```python
from build123d import *

# Parameters (mm, degrees)
AUFSATZ_LINEAR_AUSTRAGEN1_DEPTH = 15
M5_GEWINDEBOHRUNG1_D            = 4.2
M5_GEWINDEBOHRUNG1_DEPTH        = 14
M5_GEWINDEBOHRUNG1_TIP          = 1.2618073
SKIZZE4_W                       = 45
SKIZZE4_H                       = 51.25
SCHNITT_LINEAR_AUSTRAGEN1_DEPTH = 8
VERRUNDUNG1_R                   = 5
VERRUNDUNG2_R                   = 5
M3_GEWINDEBOHRUNG1_D            = 2.5
M3_GEWINDEBOHRUNG1_DEPTH        = 8.5
M3_GEWINDEBOHRUNG1_TIP          = 0.751075774


with BuildPart() as part:
    # Skizze1 → Aufsatz-Linear austragen1 (new body)
    with BuildSketch(Plane.XY):
        with BuildLine():
            Line((100.5, 0), (115, 0))
            Line((115, 0), (115, 48))
            Line((115, 48), (78.75, 84.25))
            Line((78.75, 84.25), (36.25, 84.25))
            Line((36.25, 84.25), (0, 48))
            Line((0, 48), (0, 0))
            Line((0, 0), (14.5, 0))
            Line((14.5, 0), (14.5, 23.138097353))
            ThreePointArc((14.5, 23.138097353), (14.050252532, 33.449747468), (24.361902647, 33))
            Line((24.361902647, 33), (90.638097353, 33))
            ThreePointArc((90.638097353, 33), (100.949747468, 33.449747468), (100.5, 23.138097353))
            Line((100.5, 23.138097353), (100.5, 0))
        make_face()
        with BuildLine():
            Line((68.5, 64.25), (68.5, 59.25))
            ThreePointArc((68.5, 59.25), (57.5, 48.25), (46.5, 59.25))
            Line((46.5, 59.25), (46.5, 64.25))
            ThreePointArc((46.5, 64.25), (57.5, 75.25), (68.5, 64.25))
        make_face(mode=Mode.SUBTRACT)
        with BuildLine():
            Line((43.75, 79.75), (43.75, 74.75))
            ThreePointArc((43.75, 74.75), (42, 73), (40.25, 74.75))
            Line((40.25, 74.75), (40.25, 79.75))
            ThreePointArc((40.25, 79.75), (42, 81.5), (43.75, 79.75))
        make_face(mode=Mode.SUBTRACT)
        with BuildLine():
            Line((74.75, 79.75), (74.75, 74.75))
            ThreePointArc((74.75, 74.75), (73, 73), (71.25, 74.75))
            Line((71.25, 74.75), (71.25, 79.75))
            ThreePointArc((71.25, 79.75), (73, 81.5), (74.75, 79.75))
        make_face(mode=Mode.SUBTRACT)
        with BuildLine():
            Line((74.75, 48.75), (74.75, 43.75))
            ThreePointArc((74.75, 43.75), (73, 42), (71.25, 43.75))
            Line((71.25, 43.75), (71.25, 48.75))
            ThreePointArc((71.25, 48.75), (73, 50.5), (74.75, 48.75))
        make_face(mode=Mode.SUBTRACT)
        with BuildLine():
            Line((43.75, 48.75), (43.75, 43.75))
            ThreePointArc((43.75, 43.75), (42, 42), (40.25, 43.75))
            Line((40.25, 43.75), (40.25, 48.75))
            ThreePointArc((40.25, 48.75), (42, 50.5), (43.75, 48.75))
        make_face(mode=Mode.SUBTRACT)
    extrude(amount=AUFSATZ_LINEAR_AUSTRAGEN1_DEPTH)

    # M5 Gewindebohrung1
    with Locations(Plane(origin=(0, 0, 0), x_dir=(-1, 0, 0), z_dir=(0, -1, 0))):
        with Locations((-7.5, -7.5), (-107.5, -7.5)):
            Hole(M5_GEWINDEBOHRUNG1_D / 2, depth=M5_GEWINDEBOHRUNG1_DEPTH)
            with Locations((0, 0, -(M5_GEWINDEBOHRUNG1_DEPTH + M5_GEWINDEBOHRUNG1_TIP / 2))):  # 118° drill point
                Cone(0, M5_GEWINDEBOHRUNG1_D / 2, M5_GEWINDEBOHRUNG1_TIP, mode=Mode.SUBTRACT)

    # Skizze4 → Schnitt-Linear austragen1 (cut)
    with BuildSketch(Plane(origin=(0, 0, 0), x_dir=(-1, 0, 0), z_dir=(0, 0, -1))):
        with Locations((-57.5, 58.625)):
            Rectangle(SKIZZE4_W, SKIZZE4_H)
    extrude(amount=-SCHNITT_LINEAR_AUSTRAGEN1_DEPTH, mode=Mode.SUBTRACT)

    # Verrundung1
    verrundung1_edges = [part.edges().sort_by_distance(p)[0] for p in [
        (35, 83, 4),
        (80, 83, 4),
    ]]
    fillet(verrundung1_edges, radius=VERRUNDUNG1_R)

    # Verrundung2
    verrundung2_edges = [part.edges().sort_by_distance(p)[0] for p in [
        (0, 48, 7.5),
        (36.25, 84.25, 11.5),
        (78.75, 84.25, 11.5),
        (115, 48, 7.5),
    ]]
    fillet(verrundung2_edges, radius=VERRUNDUNG2_R)

    # M3 Gewindebohrung1
    with Locations(Plane(origin=(0, 0, 0), x_dir=(-1, 0, 0), z_dir=(0, 0, -1))):
        with Locations((-3.5, 37.7), (-22.5, 37.7)):
            Hole(M3_GEWINDEBOHRUNG1_D / 2, depth=M3_GEWINDEBOHRUNG1_DEPTH)
            with Locations((0, 0, -(M3_GEWINDEBOHRUNG1_DEPTH + M3_GEWINDEBOHRUNG1_TIP / 2))):  # 118° drill point
                Cone(0, M3_GEWINDEBOHRUNG1_D / 2, M3_GEWINDEBOHRUNG1_TIP, mode=Mode.SUBTRACT)


solid = part.part
```
Model file for the job. Use its own axes, mm. A direction names the side the tool comes from. Coordinates: 2 decimals unless noted, no trailing zeros. Loops run counter-clockwise (first coordinate to the right, second up) from the corner with the lowest first, then second, coordinate; pieces in that order, holes last. Notation, with made-up numbers: (50.5, 43.25) -> (89.5, 43.25) arc R27 ccw to (89.5, 76.25) -> close; hole circle Ø6 at (61.25, -20). An arc over 180 degrees is marked (long way). Answer as a JSON object with one key per item and string values.
Q1. Pull direction Z, two halves, no side cores. Call faces 4 (the flat face through (100.5, 12, 7)), 5 (the conical face through (22.4, 37.51, 9.12)), 6 (the conical face through (107.864, 15.043, 7.484)): released by +Z, released by -Z, zero draft, split by the parting line, or undercut.
Report:
{"face 4": "zero draft", "face 5": "released by -Z", "face 6": "undercut"}
Q2. Cut at C-C (y = 28.5). List the corners of the cut face in (x, z).
Report:
{"outline": "(0, 0) -> (12, 0) -> (12, 15) -> (0, 15) -> close; (103, 0) -> (115, 0) -> (115, 15) -> (103, 15) -> close"}
Q3. Cut at A-A (x = 73). List the corners of the cut face in (y, z), and give its area (3 significant figures).
Report:
{"outline": "(33, 8) -> (42, 8) -> (42, 15) -> (33, 15) -> close; (50.5, 8) -> (73, 8) -> (73, 15) -> (50.5, 15) -> close; (81.5, 8) -> (84.25, 8) -> (84.25, 15) -> (81.5, 15) -> close", "area": "240 mm2"}
Q4. 3-axis set-ups, long thin cutter, end or side, ignore diameter. For faces 1 (the flat face through (57, 33, 9)), 2 (the flat face through (68.5, 62, 11)), 3 (the cylindrical face through (108.63, 7.1, 5.73)): which of +Z, -Z, +X, -X, +Y, -Y reach the whole face in a straight line?
Report:
{"face 1": "+Z, -Z, -Y", "face 2": "+Z, -Z", "face 3": "-Y"}
Q5. Cut at B-B (z = 3.5). List the corners of the cut face in (x, y).
Report:
{"outline": "(0, 0) -> (14.5, 0) -> (14.5, 23.14) arc R7 cw (long way) to (24.36, 33) -> (35, 33) -> (35, 70.93) arc R5 ccw to (26.46, 74.46) -> (1.46, 49.46) arc R5 ccw to (0, 45.93) -> close; (80, 33) -> (90.64, 33) arc R7 cw (long way) to (100.5, 23.14) -> (100.5, 0) -> (115, 0) -> (115, 45.93) arc R5 ccw to (113.54, 49.46) -> (88.54, 74.46) arc R5 ccw to (80, 70.93) -> close; hole circle Ø2.5 at (3.5, 37.7); hole circle Ø2.5 at (22.5, 37.7)"}
Q6. Probe probe 1 along X at (y, z) = (28.5, 7.75); probe 2 along X at (y, z) = (20, 8); probe 3 along X at (y, z) = (76, 9). List the from-to ranges inside material, lowest first.
Report:
{"probe 1": "x = 0 to 12, 103 to 115", "probe 2": "x = 0 to 14.5, 100.5 to 115", "probe 3": "x = 28 to 40.25, 43.75 to 71.25, 74.75 to 87"}
Q7. Flat gauge pins, fed straight in: P1, Ø4, axis at x = 56, y = 49, coming from the -Z side; P2, Ø4, axis at x = 18, z = 5, coming from the -Y side; P3, Ø1.5, axis at y = 77.5, z = 11, coming from the -X side. Where does each tip first touch, or does it go through?
Report:
{"P1": "stops at z = 8", "P2": "stops at y = 34.82", "P3": "stops at x = 28.75"}
Q8. Cut at D-D (z = 12.5). State how many separate pieces and enclosed holes the cut face has, and give its area (3 significant figures).
Report:
{"separate pieces": "1", "enclosed holes": "5", "area": "4,860 mm2"}
